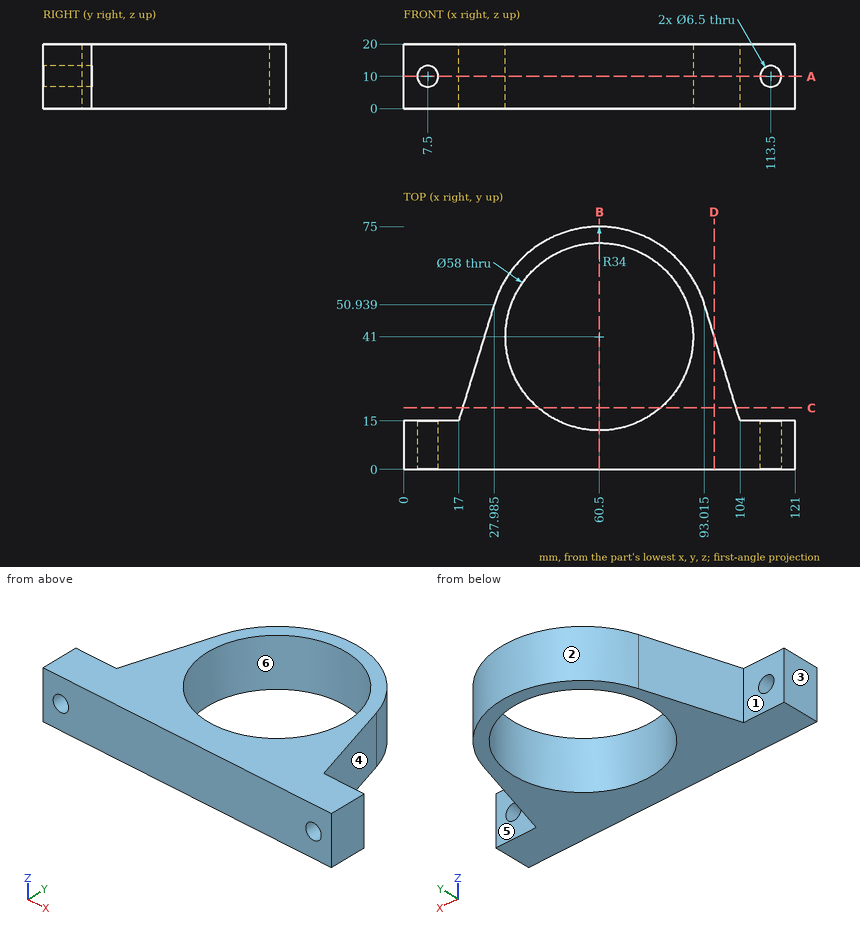
Verification items for this drawing (mm, ordinates from the low corner). A direction names the side the tool comes from. Round coordinates to 2 decimals unless told otherwise and drop trailing zeros. Loops run counter-clockwise (first coordinate to the right, second up) from the corner with the lowest first, then second, coordinate; pieces in that order, holes last. Notation, with made-up numbers: M 73,-37.5 L 122,-37.5 A29 cw 122,-3.5 Z; hole C 44.25,-17 d4. An arc over 180 degrees is marked long. Answer as a JSON object with one key per item and string values.
1. Section check B-B (x = 60.5). Record the boundary of the cut face in (y, z), plus the area to 3 significant figures.
Reply:
{"outline": "M 0,0 L 12,0 L 12,20 L 0,20 Z; M 70,0 L 75,0 L 75,20 L 70,20 Z", "area": "340 mm²"}
2. Gauge pin test, flat ends, axial feed: P1, Ø5, axis at y = 66.5, z = 8, coming from the -X side; P2, Ø2, axis at y = 17, z = 16, coming from the -X side (1 decimal); P3, Ø1.5, axis at x = 82.5, z = 12.5, coming from the +Y side. Record the tip position at first contact, or that the pin passes through.
Reply:
{"P1": "stops at x = 35.46", "P2": "stops at x = 17.3", "P3": "stops at y = 67.54"}
3. Section check C-C (y = 19). Record the boundary of the cut face in (x, z) (1 decimal).
Reply:
{"outline": "M 18.2,0 L 41.6,0 L 41.6,20 L 18.2,20 Z; M 79.4,0 L 102.8,0 L 102.8,20 L 79.4,20 Z"}
4. Section check A-A (z = 10). State how many separate pieces and enclosed holes the cut face has, plus the area to 3 significant figures.
Reply:
{"separate pieces": "3", "enclosed holes": "1", "area": "2,860 mm²"}
5. Access from +Z, -Z, +X, -X, +Y, -Y to the whole of each face (thin tool, end or side, straight path). Record for the marked faces 1 and 2.
Reply:
{"face 1": "+Z, -Z, -X, +Y", "face 2": "+Z, -Z, +Y"}
6. Section check D-D (x = 96). Record the boundary of the cut face in (y, z).
Reply:
{"outline": "M 0,0 L 41.17,0 L 41.17,20 L 0,20 Z"}
7. Scan lines: line 1 (Y direction, x = 60.5, z = 7); line 2 (Z direction, x = 7.5, y = 11); line 3 (X direction, y = 44, z = 1) (1 decimal). Record each from-to range of solid material in increasing order.
Reply:
{"line 1": "y = 0 to 12, 70 to 75", "line 2": "z = 0 to 6.75, 13.25 to 20", "line 3": "x = 25.9 to 31.7, 89.3 to 95.1"}
8. Mould release check, pull along X, two halves, no side actions. Record for the marked faces 3, 4, 5 and 6: pulls with the +X half, pulls with the -X half, needs draft (parallel to the pull), parting line crosses it, or undercut.
Reply:
{"face 3": "pulls with the -X half", "face 4": "pulls with the +X half", "face 5": "needs draft", "face 6": "undercut"}
